Answer from the drawing. Dimensions are ordinates in mm from the lowest x, y and z of the part. Coordinates: 2 decimals unless noted, no trailing zeros. Order: outer loops, then holes, each group sorted by start corner. A loop starts at its lowest first (then second) coordinate and runs counter-clockwise, first axis right, second up. Notation, with made-up numbers: (80.5, 42) - (100.5, 42) arc R16 cw to (100.5, 73) - close; hole circle Ø4 at (20, -20). An arc over 180 degrees is marked (long way). Answer as a JSON object with one key per item and string values. Group by question number.
1) Section A-A (z = 92) is taken. Give the vertices of the cut face in (x, y), plus the area to 3 significant figures.
2) Section D-D (y = 2.5) is taken. Count the separate pieces of the cut face and the enclosed holes in it, plus the area to 3 significant figures.
3) Section C-C (x = 50.5) is taken. Give the vertices of the cut face in (y, z).
4) Each of these flat-tipped pins is pushed along its axis until it touches: P1, Ø2, axis at x = 61, y = 3.5, coming from the +Z side; P2, Ø3.5, axis at x = 14.5, y = 3, coming from the +Z side; P3, Ø3, axis at y = 4, z = 99, coming from the +X side. Where does it stop, or does it pass through?
5) Find the intervals of material crossed by line 1 along X through (y, z) = (2.75, 65); line 2 along X through (y, z) = (5.5, 10.5); line 3 along X through (y, z) = (4, 97.5), in increasing order.
6) Section B-B (z = 41) is taken. Give the vertices of the cut face in (x, y).
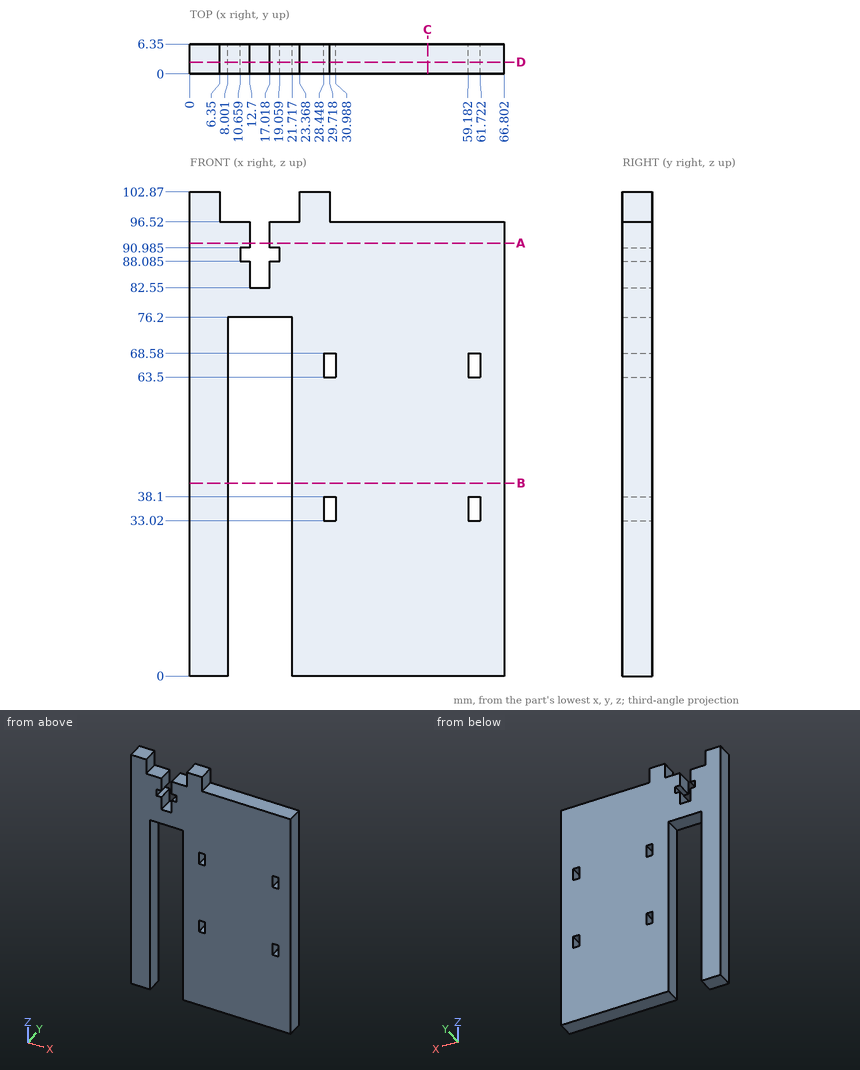
Report:
{
 "1": {"outline": "(0, 0) - (12.7, 0) - (12.7, 6.35) - (0, 6.35) - close; (17.02, 0) - (66.8, 0) - (66.8, 6.35) - (17.02, 6.35) - close", "area": "397 mm²"},
 "2": {"separate pieces": "1", "enclosed holes": "4", "area": "5,360 mm²"},
 "3": {"outline": "(0, 0) - (6.35, 0) - (6.35, 96.52) - (0, 96.52) - close"},
 "4": {"P1": "stops at z = 96.52", "P2": "stops at z = 82.55", "P3": "stops at x = 29.72"},
 "5": {"line 1": "x = 0 to 8, 21.72 to 28.45, 30.99 to 59.18, 61.72 to 66.8", "line 2": "x = 0 to 8, 21.72 to 66.8", "line 3": "x = 0 to 6.35, 23.37 to 29.72"},
 "6": {"outline": "(0, 0) - (8, 0) - (8, 6.35) - (0, 6.35) - close; (21.72, 0) - (66.8, 0) - (66.8, 6.35) - (21.72, 6.35) - close"}
}
